from build123d import *

# Parameters (mm, degrees)
SKETCH_1_W           = 39.9
SKETCH_1_H           = 20
EXTRUDE_1_DEPTH      = 1
EXTRUDE_4_DEPTH      = 19
CUT_EXTRUDE_1_DEPTH  = 13
F_3_0MM_3_AT_2_COUNT = 2
F_3_0MM_3_AT_2_PITCH = 12
EXTRUDE_5_DEPTH      = 13
CUT_EXTRUDE_2_DEPTH  = 13
SKETCH_27_R          = 1
CUT_EXTRUDE_3_DEPTH  = 6
SKETCH_28_R          = 1.5
CUT_EXTRUDE_4_DEPTH  = 26.82639154


with BuildPart() as part:
    # 草图1 → 凸台-拉伸1 (new body)
    with BuildSketch(Plane.XY):
        Rectangle(SKETCH_1_W, SKETCH_1_H)
    extrude(amount=EXTRUDE_1_DEPTH)

    # 草图2 → 凸台-拉伸4 (add)
    with BuildSketch(Plane.XY.offset(1)):
        Polygon((-19.95, 10), (-19.95, 1.025), (-14.121320344, 1.025), (-12, 3.146320344), (0, 3.146320344), (0, 10), align=None)
        Polygon((19.95, 10), (0, 10), (0, 3.146320344), (12, 3.146320344), (14.121320344, 1.025), (19.95, 1.025), align=None)
        Polygon((-8, -1.75), (-10.5, 1.75), (-2.5, 1.75), (-2.5, -1.75), align=None)
        Polygon((2.5, -1.75), (2.5, 1.75), (10.5, 1.75), (8, -1.75), align=None)
        Polygon((-12.45, -1.025), (-19.95, -1.025), (-19.95, -10), (19.95, -10), (19.95, -1.025), (12.45, -1.025), (10.646428571, -3.55), (-10.646428571, -3.55), align=None)
    extrude(amount=EXTRUDE_4_DEPTH)

    # 草图4 → 切除-拉伸1 (cut)
    with BuildSketch(Plane.XY.offset(20)):
        Polygon((-12.45, -1.025), (-11.193517665, -10), (0, -13.387486255), (11.193517665, -10), (12.45, -1.025), (10.646428571, -3.55), (-10.646428571, -3.55), align=None)
        Polygon((-14.121320344, 1.025), (-12.45, 12.563933046), (12.45, 12.563933046), (14.121320344, 1.025), (12, 3.146320344), (-12, 3.146320344), align=None)
    extrude(amount=-CUT_EXTRUDE_1_DEPTH, mode=Mode.SUBTRACT)

    # 草图22 → Ø3.0mm 暗销孔3 (revolve, cut)
    with BuildSketch(Plane(origin=(-15.5, -10, 16), x_dir=(0, 0, -1), z_dir=(1, 0, 0))):
        Polygon((0, 0), (0, 6.901290929), (1.5, 6), (1.5, 0), align=None)
    f_3_0mm_3 = revolve(axis=Axis((-15.5, -16.35, 16), (0, 1, 0)), mode=Mode.SUBTRACT)

    # Ø3.0mm 暗销孔3 at 2: Ø3.0mm 暗销孔3 ×2
    with Locations(*[(0, 0, -i * F_3_0MM_3_AT_2_PITCH) for i in range(1, F_3_0MM_3_AT_2_COUNT)]):
        add(f_3_0mm_3, mode=Mode.SUBTRACT)

    # 镜向3: Ø3.0mm 暗销孔3 across plane
    add(f_3_0mm_3.mirror(Plane(origin=(0, 0, 0), x_dir=(0, 0, 1), z_dir=(1, 0, 0))), mode=Mode.SUBTRACT)

    # 镜向3 copy 1 sketch → 镜向3 copy 1 (revolve, cut)
    with BuildSketch(Plane(origin=(15.5, -10, 4), x_dir=(0, 0, -1), z_dir=(-1, 0, 0))):
        Polygon((0, 0), (0, -6.901290929), (1.5, -6), (1.5, 0), align=None)
    revolve(axis=Axis((15.5, -16.35, 4), (0, -1, 0)), mode=Mode.SUBTRACT)

    # 草图25 → 凸台-拉伸5 (add)
    with BuildSketch(Plane.XY.offset(7)):
        Polygon((-12.821364791, 10), (-12, 3.146320344), (-14.121320344, 1.025), align=None)
        Polygon((12, 3.146320344), (14.121320344, 1.025), (12.821364791, 10), align=None)
    extrude(amount=EXTRUDE_5_DEPTH)

    # 草图26 → 切除-拉伸2 (cut)
    with BuildSketch(Plane.XY.offset(20)):
        Polygon((-11.872508119, -5.15), (-11.872508119, -10), (-11.193517665, -10), align=None)
        Polygon((11.193517665, -10), (11.872508119, -5.15), (11.872508119, -10), align=None)
    extrude(amount=-CUT_EXTRUDE_2_DEPTH, mode=Mode.SUBTRACT)

    # 草图27 → 切除-拉伸3 (cut)
    with BuildSketch(Plane.XY.offset(20)):
        with Locations((-16.2, 5.5)):
            Circle(SKETCH_27_R)
        with Locations(Location((16.2, 5.5, 0), (0, 0, 180))):
            Circle(SKETCH_27_R)
    extrude(amount=-CUT_EXTRUDE_3_DEPTH, mode=Mode.SUBTRACT)

    # 草图28 → 切除-拉伸4 (cut, through all)
    with BuildSketch(Plane.XY.offset(7)):
        with Locations((-8, 7.5)):
            Circle(SKETCH_28_R)
        with Locations((-8, -7.5)):
            Circle(SKETCH_28_R)
        with Locations(Location((8, -7.5, 0), (0, 0, 180))):
            Circle(SKETCH_28_R)
        with Locations(Location((8, 7.5, 0), (0, 0, 180))):
            Circle(SKETCH_28_R)
    extrude(amount=-CUT_EXTRUDE_4_DEPTH, mode=Mode.SUBTRACT)


solid = part.part
Could you check a few things on this model? Use its own coordinates, in mm. A direction names the side the tool comes from. Give positions to 0.01 mm unless a question says otherwise; leave off trailing zeros. Order: outer loops, then holes, each group sorted by start corner. A loop starts at its lowest first (then second) coordinate and runs counter-clockwise, first axis right, second up. Notation, with made-up numbers: (51.25, 6.25) -> (77.25, 6.25) arc R14 ccw to (77.25, 11.25) -> close; hole circle Ø3 at (-38, 53.25). An arc over 180 degrees is marked (long way). Answer in a Markdown table with one row per item. Add a question column.
Item 1: Imagine slicing it at D-D (y = 8.25). List the corners of the cut face in (x, z) for me, and give its area (3 significant figures).
Item 2: I'm going to push flat-ended pins straight in: P1, Ø0.6, axis at x = -16.5, y = 5.5, coming from the +Z side; P2, Ø7.5, axis at x = 4, y = 7, coming from the +Z side; P3, Ø2.5, axis at x = -8, y = 7.5, coming from the +Z side; P4, Ø1.8, axis at x = -15.5, z = 4, coming from the -Y side. Where does each tip first touch, or does it pass through?
Item 3: For faces 1 (the flat face through (-17, 1.025, 10)), 2 (the flat face through (-12.416, 6.621, 13.409)), 3 (the flat face through (16, 5, 14)), which set-ups out of +Z, -Z, +X, -X, +Y, -Y let a thin tool reach every point of the face, with its end or its side?
Item 4: Imagine slicing it at A-A (z = 2). List the corners of the cut face in (x, y) for me (3 decimals).
Item 5: We'd pull the mould along X, two halves only. Please class faces 4 (the flat face through (0, 0, 0)), 5 (the flat face through (-9.232, -0.024, 10.367)): pulls with the +X half, pulls with the -X half, needs draft (parallel to the pull), parting line crosses it, or undercut.
Item 6: Please list where these lines run through material, in increasing order: probe 1 along X at (y, z) = (-5.25, 4); probe 2 along Y at (x, z) = (-16.2, 18.3) (3 decimals); probe 3 along Y at (x, z) = (-3, 2).
Item 7: Imagine slicing it at C-C (x = -1.5). List the corners of the cut face in (y, z) for me, and give its area (3 significant figures).
Item 8: Imagine slicing it at B-B (y = -6.75). List the corners of the cut face in (x, z) for me, and give its area (3 significant figures).
Result:
| question | item | result |
|---|---|---|
| 1 | outline | (-19.95, 0) -> (-9.3, 0) -> (-9.3, 7) -> (-12.61, 7) -> (-12.61, 20) -> (-19.95, 20) -> close; (-6.7, 0) -> (6.7, 0) -> (6.7, 7) -> (-6.7, 7) -> close; (9.3, 0) -> (19.95, 0) -> (19.95, 20) -> (12.61, 20) -> (12.61, 7) -> (9.3, 7) -> close |
| 1 | area | 434 mm2 |
| 2 | P1 | z = 14 |
| 2 | P2 | z = 7 |
| 2 | P3 | through |
| 2 | P4 | y = -3.64 |
| 3 | face 1 | +Z, -X |
| 3 | face 2 | +Z, +Y |
| 3 | face 3 | +Z |
| 4 | outline | (-19.95, -10) -> (19.95, -10) -> (19.95, -1.025) -> (12.45, -1.025) -> (10.646, -3.55) -> (-10.646, -3.55) -> (-12.45, -1.025) -> (-19.95, -1.025) -> close; (-19.95, 1.025) -> (-14.121, 1.025) -> (-12, 3.146) -> (12, 3.146) -> (14.121, 1.025) -> (19.95, 1.025) -> (19.95, 10) -> (-19.95, 10) -> close; (-10.5, 1.75) -> (-8, -1.75) -> (-2.5, -1.75) -> (-2.5, 1.75) -> close; (2.5, -1.75) -> (8, -1.75) -> (10.5, 1.75) -> (2.5, 1.75) -> close; hole circle Ø3 at (-8, -7.5); hole circle Ø3 at (-8, 7.5); hole circle Ø3 at (8, -7.5); hole circle Ø3 at (8, 7.5) |
| 5 | face 4 | needs draft |
| 5 | face 5 | undercut |
| 6 | probe 1 | -19.95 to -17, -14 to 14, 17 to 19.95 |
| 6 | probe 2 | -10 to -1.025, 1.025 to 4.5, 6.5 to 10 |
| 6 | probe 3 | -10 to -3.55, -1.75 to 1.75, 3.15 to 10 |
| 7 | outline | (-10, 0) -> (10, 0) -> (10, 7) -> (3.15, 7) -> (3.15, 1) -> (-3.55, 1) -> (-3.55, 7) -> (-10, 7) -> close |
| 7 | area | 99.8 mm2 |
| 8 | outline | (-19.95, 0) -> (-9.3, 0) -> (-9.3, 7) -> (-11.87, 7) -> (-11.87, 20) -> (-19.95, 20) -> close; (-6.7, 0) -> (6.7, 0) -> (6.7, 7) -> (-6.7, 7) -> close; (9.3, 0) -> (19.95, 0) -> (19.95, 20) -> (11.87, 20) -> (11.87, 7) -> (9.3, 7) -> close; hole circle Ø3 at (-15.5, 4); hole circle Ø3 at (-15.5, 16); hole circle Ø3 at (15.5, 4); hole circle Ø3 at (15.5, 16) |
| 8 | area | 425 mm2 |
